Here's how the part is built. I have some questions about the finished solid (model axes, mm). Face numbers are marked on the shaded views. Round coordinates to 2 decimals unless told otherwise and drop trailing zeros. Write each loop counter-clockwise with the first axis right and the second up, starting at its lowest first coordinate (ties: lowest second). Pieces come first, ordered by that corner, then holes. Notation, with made-up numbers: (66, 34) - (70, 34) arc R25 ccw to (70, 53) - close; hole circle Ø10 at (42, 1). An arc over 180 degrees is marked (long way). Write item = value, one per line. Start each with the question number.
Item 1: If we section it at B-B (z = -4.3): Please give me the cut outline in (x, y).
Item 2: For P1, Ø10.5, axis at x = 18.05, y = 6.125, coming from the -Z side; P2, Ø6, axis at x = 53.5, z = -3.5, coming from the +Y side; P3, Ø4, axis at x = 60, z = -5, coming from the -Y side, each with a flat end and sliding along its axis, tell me the tip position at first contact or that it passes through.
Item 3: If I drill on line 1 along Y through (x, z) = (43.45, 0.8) (3 decimals); line 2 along Y through (x, z) = (18.05, 1.35) (3 decimals); line 3 along X through (y, z) = (-33.5, 0.5), over which ranges is the centre line in solid material (lowest first)? Write a range as [from, to].
Item 4: If we section it at D-D (x = 43.45): Please give me the cut outline in (y, z) (3 decimals), and give its area (3 significant figures).
Item 5: If we section it at A-A (y = -42.5): Please give me the cut outline in (x, z) (3 decimals).
Item 6: If we section it at C-C (x = 18.05): Please give me the cut outline in (y, z) (3 decimals).
Item 7: Thinking about a two-plate mould opening in Y: for the marked faces 1 and 2, which applies, pulls with the +Y half, pulls with the -Y half, needs draft (parallel to the pull), parting line crosses it, or undercut?
```python
from build123d import *

# Parameters (mm, degrees)
SKETCH1_W           = 55
SKETCH1_H           = 100
SKETCH1_W_2         = 27.5
SKETCH1_H_2         = 22
BOSS_EXTRUDE1_DEPTH = 3.175
SKETCH2_W           = 8
SKETCH2_H           = 60
BOSS_EXTRUDE2_DEPTH = 10
SKETCH3_W           = 8
SKETCH3_H           = 45
CUT_EXTRUDE1_DEPTH  = 10
SKETCH4_R           = 1.5
CUT_EXTRUDE2_DEPTH  = 119.348003785
SKETCH5_R           = 3.25
CUT_EXTRUDE3_DEPTH  = 108.993055332
SKETCH7_W           = 8
SKETCH7_H           = 45
CUT_EXTRUDE5_DEPTH  = 108.993055332
SKETCH8_W           = 3.175
SKETCH8_H           = 10
BOSS_EXTRUDE4_DEPTH = 8
SKETCH9_R           = 1.025
CUT_EXTRUDE6_DEPTH  = 108.993055332


with BuildPart() as part:
    # Sketch1 → Boss-Extrude1 (new body)
    with BuildSketch(Plane.XY):
        with Locations((35, -37.5)):
            Rectangle(SKETCH1_W, SKETCH1_H)
        with Locations((36.25, -37.5)):
            Rectangle(SKETCH1_W_2, SKETCH1_H_2, mode=Mode.SUBTRACT)
    extrude(amount=BOSS_EXTRUDE1_DEPTH)

    # Sketch2 → Boss-Extrude2 (add)
    with BuildSketch(Plane(origin=(0, 0, 0), x_dir=(-1, 0, 0), z_dir=(0, 0, -1))):
        with Locations((-58.5, -37.5)):
            Rectangle(SKETCH2_W, SKETCH2_H)
    extrude(amount=BOSS_EXTRUDE2_DEPTH)

    # Sketch3 → Cut-Extrude1 (cut)
    with BuildSketch(Plane(origin=(0, 0, -10), x_dir=(-1, 0, 0), z_dir=(0, 0, -1))):
        with Locations((-58.5, -37.5)):
            Rectangle(SKETCH3_W, SKETCH3_H)
    extrude(amount=-CUT_EXTRUDE1_DEPTH, mode=Mode.SUBTRACT)

    # Sketch4 → Cut-Extrude2 (cut, through all)
    with BuildSketch(Plane(origin=(0, 12.5, 0), x_dir=(1, 0, 0), z_dir=(0, 1, 0))):
        with Locations(Location((58.5, 4.3, 0), (0, 0, 270))):
            Circle(SKETCH4_R)
    extrude(amount=-CUT_EXTRUDE2_DEPTH, mode=Mode.SUBTRACT)

    # Sketch5 → Cut-Extrude3 (cut, through all)
    with BuildSketch(Plane(origin=(0, 0, 0), x_dir=(-1, 0, 0), z_dir=(0, 0, -1))):
        with Locations((-43.45, -81.125)):
            Circle(SKETCH5_R)
        with Locations((-18.05, -81.125)):
            Circle(SKETCH5_R)
        with Locations((-18.05, 6.125)):
            Circle(SKETCH5_R)
        with Locations((-43.45, 6.125)):
            Circle(SKETCH5_R)
    extrude(amount=-CUT_EXTRUDE3_DEPTH, mode=Mode.SUBTRACT)

    # Sketch7 → Cut-Extrude5 (cut, through all)
    with BuildSketch(Plane(origin=(0, 0, 0), x_dir=(-1, 0, 0), z_dir=(0, 0, -1))):
        with Locations((-58.5, -37.5)):
            Rectangle(SKETCH7_W, SKETCH7_H)
    extrude(amount=-CUT_EXTRUDE5_DEPTH, mode=Mode.SUBTRACT)

    # Sketch8 → Boss-Extrude4 (add)
    with BuildSketch(Plane(origin=(54.5, 0, 0), x_dir=(0, 0, -1), z_dir=(1, 0, 0))):
        with Locations((-1.5875, -42.5)):
            Rectangle(SKETCH8_W, SKETCH8_H)
    extrude(amount=BOSS_EXTRUDE4_DEPTH)

    # Sketch9 → Cut-Extrude6 (cut, through all)
    with BuildSketch(Plane(origin=(0, 0, 0), x_dir=(-1, 0, 0), z_dir=(0, 0, -1))):
        with Locations((-54.7, -42.5)):
            Circle(SKETCH9_R)
    extrude(amount=-CUT_EXTRUDE6_DEPTH, mode=Mode.SUBTRACT)


solid = part.part
```
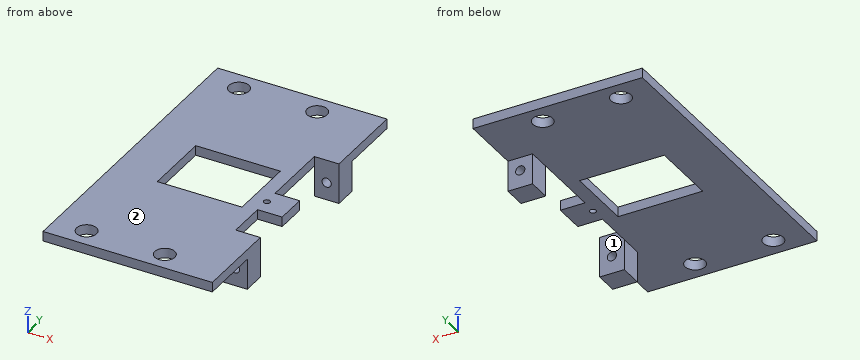
Reply:
q1.outline = (54.5, -67.5) - (57, -67.5) - (57, -60) - (54.5, -60) - close; (54.5, -15) - (57, -15) - (57, -7.5) - (54.5, -7.5) - close; (60, -67.5) - (62.5, -67.5) - (62.5, -60) - (60, -60) - close; (60, -15) - (62.5, -15) - (62.5, -7.5) - (60, -7.5) - close
q2.P1 = 0
q2.P2 = -7.5
q2.P3 = -67.5
q3.line_1 = [-87.5, -84.375], [-77.875, -48.5], [-26.5, 2.875], [9.375, 12.5]
q3.line_2 = [-87.5, -84.375], [-77.875, 2.875], [9.375, 12.5]
q3.line_3 = [7.5, 22.5], [50, 54.5]
q4.outline = (-87.5, 0) - (-84.375, 0) - (-84.375, 3.175) - (-87.5, 3.175) - close; (-77.875, 0) - (-48.5, 0) - (-48.5, 3.175) - (-77.875, 3.175) - close; (-26.5, 0) - (2.875, 0) - (2.875, 3.175) - (-26.5, 3.175) - close; (9.375, 0) - (12.5, 0) - (12.5, 3.175) - (9.375, 3.175) - close
q4.area = 206 mm2
q5.outline = (7.5, 0) - (22.5, 0) - (22.5, 3.175) - (7.5, 3.175) - close; (50, 0) - (53.675, 0) - (53.675, 3.175) - (50, 3.175) - close; (55.725, 0) - (62.5, 0) - (62.5, 3.175) - (55.725, 3.175) - close
q6.outline = (-87.5, 0) - (-84.375, 0) - (-84.375, 3.175) - (-87.5, 3.175) - close; (-77.875, 0) - (2.875, 0) - (2.875, 3.175) - (-77.875, 3.175) - close; (9.375, 0) - (12.5, 0) - (12.5, 3.175) - (9.375, 3.175) - close
q7.face_1 = undercut
q7.face_2 = needs draft
